Autodesk Inventor part; units mm, degrees
ref_plane "YZ Plane" through (0, 0, 0) normal (1, 0, 0) x (0, 1, 0)
ref_plane "XZ Plane" through (0, 0, 0) normal (0, 1, 0) x (-1, 0, 0)
ref_plane "XY Plane" through (0, 0, 0) normal (0, 0, 1) x (1, 0, 0)
sketch "Sketch1" plane through (0, 0, 0) normal (0, 1, 0) x (-1, 0, 0)
  line L0 (0, 0) -> (20, 0)
  line L1 (20, 0) -> (20, -86)
  line L2 (20, -86) -> (0, -86)
  line L3 (0, -86) -> (0, 0)
  dimension "d0" = 20
  dimension "d1" = 86
extrude "Extrusion1" add sketch "Sketch1" along normal blind 2
sketch "Sketch2" plane through (0, 2, 0) normal (0, 1, 0) x (1, 0, 0)
  line L0 (0, 0) -> (0, 86)
  line L1 (0, 0) -> (-11.5, 0)
  line L2 (-20, 0) -> (0, 0)
  line L3 (-11.5, -3.5) -> (-11.5, 3.5) construction
  line L4 (-9.5, -3.5) -> (-9.5, 3.5)
  line L5 (-13.5, 3.5) -> (-13.5, -3.5)
  arc A0 (-13.5, -3.5) -> (-9.5, -3.5) centre (-11.5, -3.5) ccw
  arc A1 (-9.5, 3.5) -> (-13.5, 3.5) centre (-11.5, 3.5) ccw
  line L6 (-11.5, 89.5) -> (-11.5, 82.5) construction
  line L7 (0, 86) -> (-20, 86)
  line L8 (-13.5, 89.5) -> (-13.5, 82.5)
  line L9 (-9.5, 82.5) -> (-9.5, 89.5)
  arc A2 (-9.5, 89.5) -> (-13.5, 89.5) centre (-11.5, 89.5) ccw
  arc A3 (-13.5, 82.5) -> (-9.5, 82.5) centre (-11.5, 82.5) ccw
  line L10 (-11.5, 86) -> (-4.5, 86) construction
  dimension "d4" = 11.5
  dimension "d5" = 3.5
  dimension "d6" = 4
  dimension "d7" = 3.5
  dimension "d8" = 90
  dimension "d9" = 4
  dimension "d10" = 11.5
extrude "Extrusion2" cut sketch "Sketch2" against normal blind 2
sketch "Sketch3" plane through (0, 2, 0) normal (0, 1, 0) x (1, 0, 0)
  arc A0 (-9.5, 3.5) -> (-13.5, 3.5) centre (-11.5, 3.5) ccw
  line L0 (-11.5, 3.5) -> (-11.5, 6.5)
  arc A1 (-13.5, 82.5) -> (-9.5, 82.5) centre (-11.5, 82.5) ccw
  line L1 (-11.5, 82.5) -> (-11.5, 79.5)
  line L2 (-11.5, 79.5) -> (-20, 79.5)
  line L3 (-20, 0) -> (-20, 86)
  line L4 (-11.5, 6.5) -> (-2, 6.5)
  line L5 (0, 86) -> (0, 0)
  line L6 (-2, 6.5) -> (-20, 6.5)
  line L7 (-20, 6.5) -> (-20, 79.5)
  line L8 (-20, 79.5) -> (-2, 79.5)
  line L9 (-2, 79.5) -> (-2, 6.5)
  dimension "d13" = 3
  dimension "d14" = 3
  dimension "d15" = 9.5
extrude "Extrusion3" add sketch "Sketch3" along normal blind 53
properties part number "DM332T_Stepper"
Source: CAD feature listing. Evaluate the final solid. Frame: model axes, mm. A direction names the side the tool comes from. Round coordinates to 2 decimals unless told otherwise and drop trailing zeros. Loops run counter-clockwise (first coordinate to the right, second up) from the corner with the lowest first, then second, coordinate; pieces in that order, holes last. Notation, with made-up numbers: (-1, 73.25) - (25, 73.25) arc R22 cw to (25, 100.25) - close; hole circle Ø10 at (71, 81.5). An arc over 180 degrees is marked (long way). Write item = value, one per line. Start each with the question number.
(1) Pull-direction query (X, two-part tool) for faces 1 (the face through (-5, 1, 0)), 2 (the face through (-13.5, 1, -84)), 3 (the face through (-2, 28, -44)); classes: +X half, -X half, draft (parallel to the pull), parting line (faces both ways), or undercut.
(2) Section query C-C, the plane y = 39. Output: boundary loops of the cut face in (x, z).
(3) Section query A-A, the plane x = -11.5. Output: boundary loops of the cut face in (y, z), plus the area to 3 significant figures.
(4) Section query B-B, the plane z = -14. Output: boundary loops of the cut face in (x, y).
(5) Ray query, line 1 along Z through (x, y) = (-12.25, 51); line 2 along X through (y, z) = (46, -37.5); line 3 along Y through (x, z) = (-1, -9). Return the intervals inside material, ascending. Write a range as from..to.
(6) Set-up query: faces 4 (the face through (-13.5, 1, -2)), 5 (the face through (-9.5, 1, -84)), 6 (the face through (-11, 28, -79.5)), 7 (the face through (-11, 28, -6.5)). Return all of +Z, -Z, +X, -X, +Y, -Y with unobstructed straight access to the full face (end or side cutting, diameter ignored); none if empty.
(7) Pin query (flat end, axial travel): pin 1 (9 mm diameter, centred on x = -15, y = 22, fed in from +Z); pin 2 (10 mm diameter, centred on y = 34.5, z = -62.5, fed in from +X). Return the tip coordinate at first contact, or that it passes through.
Conclusion:
q1.face_1 = draft
q1.face_2 = undercut
q1.face_3 = +X half
q2.outline = (-20, -79.5) - (-2, -79.5) - (-2, -6.5) - (-20, -6.5) - close
q3.outline = (0, -80.5) - (2, -80.5) - (2, -79.5) - (55, -79.5) - (55, -6.5) - (2, -6.5) - (2, -5.5) - (0, -5.5) - close
q3.area = 4,020 mm2
q4.outline = (-20, 0) - (0, 0) - (0, 2) - (-2, 2) - (-2, 55) - (-20, 55) - close
q5.line_1 = -79.5..-6.5
q5.line_2 = -20..-2
q5.line_3 = 0..2
q6.face_4 = +Z, +Y, -Y
q6.face_5 = -Z, +Y, -Y
q6.face_6 = -Z, +X, -X, +Y
q6.face_7 = +Z, +X, -X, +Y
q7.pin_1 = -6.5
q7.pin_2 = -2
